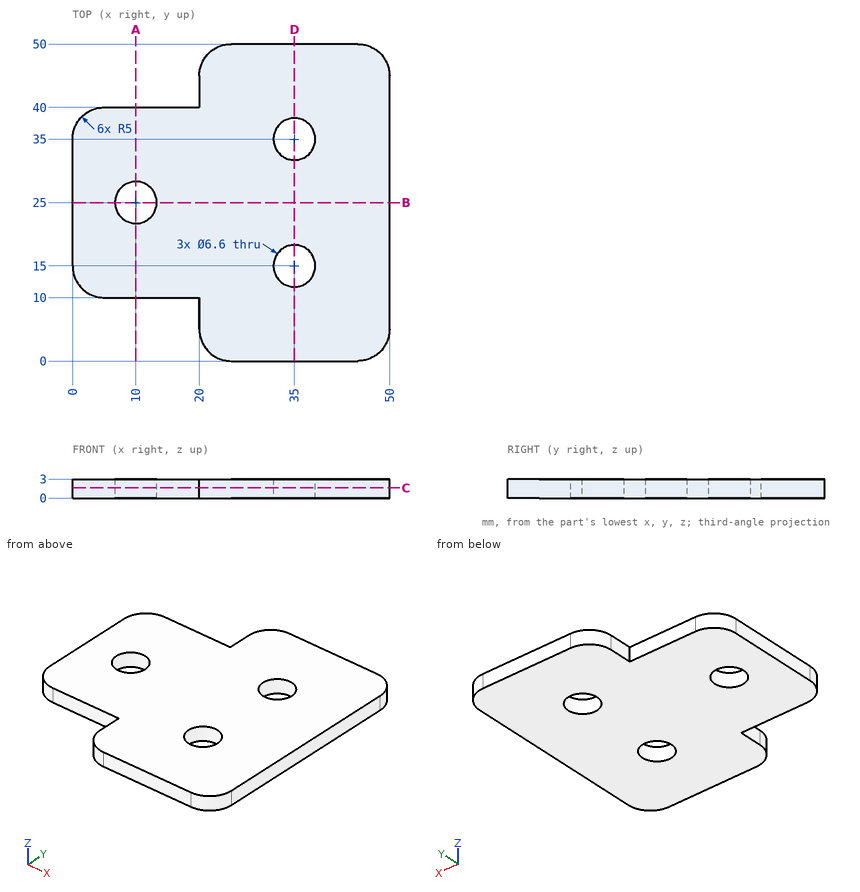
Job drawing, mm, ordinate dimensions from the low corner. One solid piece. Round coordinates to 2 decimals unless told otherwise and drop trailing zeros. Order: outer loops, then holes, each group sorted by start corner. A loop starts at its lowest first (then second) coordinate and runs counter-clockwise, first axis right, second up. Notation, with made-up numbers: (-12.75, 46) -> (39.25, 46) arc R38 cw to (39.25, 84) -> close; hole circle Ø10 at (17, 9.5). An arc over 180 degrees is marked (long way). Answer in a Markdown table with one row per item.
1) Wall check: L1, parallel to Y at x = 35, z = 0.85; L2, parallel to Y at x = 10, z = 0.75; L3, parallel to Y at x = 6, z = 0.25. Give the ranges that are in metal, low to high.
Values:
| item | result |
|---|---|
| L1 | 0 to 11.7, 18.3 to 31.7, 38.3 to 50 |
| L2 | 10 to 21.7, 28.3 to 40 |
| L3 | 10 to 40 |
2) Band-saw the part on D-D on x = 35. Give the cut face in (y, z), and give its area (3 significant figures).
Values:
| item | result |
|---|---|
| outline | (0, 0) -> (11.7, 0) -> (11.7, 3) -> (0, 3) -> close; (18.3, 0) -> (31.7, 0) -> (31.7, 3) -> (18.3, 3) -> close; (38.3, 0) -> (50, 0) -> (50, 3) -> (38.3, 3) -> close |
| area | 110 mm2 |
3) Band-saw the part on C-C on z = 1.6. Give the cut face in (x, y).
Values:
| item | result |
|---|---|
| outline | (0, 15) arc R5 ccw to (5, 10) -> (20, 10) -> (20, 5) arc R5 ccw to (25, 0) -> (45, 0) arc R5 ccw to (50, 5) -> (50, 45) arc R5 ccw to (45, 50) -> (25, 50) arc R5 ccw to (20, 45) -> (20, 40) -> (5, 40) arc R5 ccw to (0, 35) -> close; hole circle Ø6.6 at (10, 25); hole circle Ø6.6 at (35, 15); hole circle Ø6.6 at (35, 35) |
4) Pin check, flat tip, straight feed: P1, Ø0.9, axis at y = 42, z = 1.5, coming from the -X side. Stop position of the tip, or through.
Values:
| item | result |
|---|---|
| P1 | x = 20 |
5) Band-saw the part on A-A on x = 10. Give the cut face in (y, z).
Values:
| item | result |
|---|---|
| outline | (10, 0) -> (21.7, 0) -> (21.7, 3) -> (10, 3) -> close; (28.3, 0) -> (40, 0) -> (40, 3) -> (28.3, 3) -> close |
6) Band-saw the part on B-B on y = 25. Give the cut face in (x, z), and give its area (3 significant figures).
Values:
| item | result |
|---|---|
| outline | (0, 0) -> (6.7, 0) -> (6.7, 3) -> (0, 3) -> close; (13.3, 0) -> (50, 0) -> (50, 3) -> (13.3, 3) -> close |
| area | 130 mm2 |
